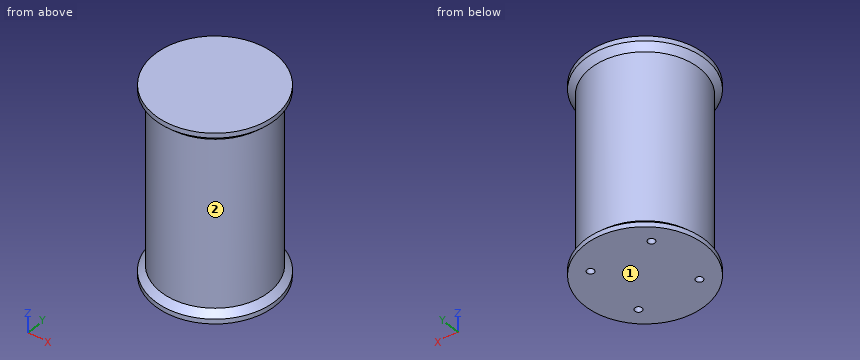
Autodesk Inventor part; units mm, degrees
ref_plane "YZ Plane" through (0, 0, 0) normal (1, 0, 0) x (0, 1, 0)
ref_plane "XZ Plane" through (0, 0, 0) normal (0, 1, 0) x (-1, 0, 0)
ref_plane "XY Plane" through (0, 0, 0) normal (0, 0, 1) x (1, 0, 0)
sketch "Sketch1" plane through (0, 0, 0) normal (0, 0, 1) x (1, 0, 0)
  circle A0 centre (0, 0) radius 22.5
  point P0 (-12.5, 12.5)
  point P1 (12.5, 12.5)
  point P2 (12.5, -12.5)
  point P3 (-12.5, -12.5)
  dimension "d0" = 45
  dimension "d1" = 25
  dimension "d2" = 25
  dimension "d3" = 12.5
  dimension "d4" = 12.5
extrude "Extrusion1" add sketch "Sketch1" along normal blind 75
sketch "Sketch2" plane through (0, 0, 75) normal (0, 0, 1) x (1, 0, 0)
  circle A0 centre (0, 0) radius 22.5
  circle A1 centre (0, 0) radius 25
  dimension "d7" = 2.5
extrude "Extrusion2" add sketch "Sketch2" along normal blind 2 contours A0 | A1
chamfer "Chamfer1" distance 2.5 angle 45 1 edges at (-22.5, 0, 75)
sketch "Sketch3" plane through (0, 0, 0) normal (0, 0, -1) x (-1, 0, 0)
  circle A0 centre (0, 0) radius 25
extrude "Extrusion3" add sketch "Sketch3" along normal blind 2
chamfer "Chamfer2" distance 2.5 angle 45 1 edges at (-22.5, 0, 0)
sketch "Sketch4" plane through (0, 0, -2) normal (0, 0, -1) x (-1, 0, 0)
  circle A0 centre (0, 0) radius 25
  point P0 (-12.5, 12.5)
  point P1 (12.5, 12.5)
  point P2 (12.5, -12.5)
  point P3 (-12.5, -12.5)
  dimension "d18" = 12.5
  dimension "d19" = 12.5
  dimension "d20" = 12.5
  dimension "d21" = 12.5
hole "Hole1" at (12.5, 12.5, -2) at (-12.5, 12.5, -2) at (-12.5, -12.5, -2) at (12.5, -12.5, -2) direction (0, 0, 1) diameter 2.9 depth 20 tip angle 118
properties part number "Filament Spool Holder" material "ABS Plastic"
Work out the finished part from the listing and answer in its coordinate system (mm). Face numbers are marked on the shaded views. Give positions to 0.01 mm unless a question says otherwise; leave off trailing zeros. Loops run counter-clockwise (first coordinate to the right, second up) from the corner with the lowest first, then second, coordinate; pieces in that order, holes last. Notation, with made-up numbers: (3, 25.25) - (62, 25.25) arc R27 ccw to (62, 54.25) - close; hole circle Ø10 at (72, -24.5). An arc over 180 degrees is marked (long way). Answer in a Markdown table with one row per item.
(1) Flat-ended cylindrical pins translate along their axes: pin 1 Ø8 at (x, z) = (-15.5, 68) entering from +Y; pin 2 Ø6 at (y, z) = (18.5, 25.5) entering from +X; pin 3 Ø3 at (y, z) = (-12, 60.5) entering from -X. Find the tip coordinate at first contact, or state that the pin passes through.
Results list:
| item | result |
|---|---|
| pin 1 | stops at y = 19.34 |
| pin 2 | stops at x = 16.31 |
| pin 3 | stops at x = -19.9 |
(2) Section C-C (z = 4) is taken. Give the vertices of the cut face in (x, y).
Results list:
| item | result |
|---|---|
| outline | circle Ø45 at (0, 0); hole circle Ø2.9 at (-12.5, -12.5); hole circle Ø2.9 at (-12.5, 12.5); hole circle Ø2.9 at (12.5, -12.5); hole circle Ø2.9 at (12.5, 12.5) |
(3) Section D-D (z = 47) is taken. Give the vertices of the cut face in (x, y), and give its area (3 significant figures).
Results list:
| item | result |
|---|---|
| outline | circle Ø45 at (0, 0) |
| area | 1,590 mm² |
(4) For a pull along Y with two mould halves and no side action, classify the marked faces 1 and 2 as pulls with the +Y half, pulls with the -Y half, needs draft (parallel to the pull), parting line crosses it, or undercut.
Results list:
| item | result |
|---|---|
| face 1 | needs draft |
| face 2 | parting line crosses it |
(5) Consider L1, parallel to Y at x = -12, z = 5; L2, parallel to Y at x = -12.5, z = 8.25. Determine where each line is inside the solid, lowest interval first. Write a range as [from, to].
Results list:
| item | result |
|---|---|
| L1 | y = [-19.03, -13.86], [-11.14, 11.14], [13.86, 19.03] |
| L2 | y = [-18.71, -13.95], [-11.05, 11.05], [13.95, 18.71] |
